The model under review builds one solid part; all positions refer to its coordinate system, in mm. A direction names the side the tool comes from. Round coordinates to 2 decimals unless told otherwise and drop trailing zeros. Write each loop counter-clockwise with the first axis right and the second up, starting at its lowest first coordinate (ties: lowest second). Pieces come first, ordered by that corner, then holes. Notation, with made-up numbers: (51, 79) -> (66, 79) arc R27 ccw to (66, 111) -> close; hole circle Ø3 at (82, 55). An arc over 180 degrees is marked (long way). Return JSON: item names as keys, results as strings. Group by question number.
1. Take a section at C-C, the plane y = -63. Write out the cut boundary in (x, z).
2. Take a section at B-B, the plane x = 33.5. Write out the cut boundary in (y, z), then the cut area to 3 significant figures.
3. Mouldability with a two-part tool opening along X and no side actions: class faces 1 (the flat face through (31, -38, 8.113)), 2 (the flat face through (53, -65, 33.513)), 3 (the flat face through (60.477, -47, 2)) as pulls with the +X half, pulls with the -X half, needs draft (parallel to the pull), parting line crosses it, or undercut.
4. Take a section at A-A, the plane z = 11.5. Write out the cut boundary in (x, y), then the cut area to 3 significant figures.
5. For line 1 along Z through (x, y) = (34, -16.5); line 2 along X through (y, z) = (-61, 18.5); line 3 along Y through (x, z) = (43, 29.5), list the stretches that pass through material, from the lowest coordinate up. Write a range as from..to.
6. Take a section at D-D, the plane x = -11.5. Write out the cut boundary in (y, z).
7. Tool access review of faces 4 (the flat face through (3.45, -38.63, 20.63)), 5 (the flat face through (47.955, -56.883, 20.635)), 6 (the flat face through (-1, 0, 8)): name each direction out of +Z, -Z, +X, -X, +Y, -Y from which nothing blocks a thin tool from reaching the whole face with its end or side.
8. Clearance check with a flat-ended pin moving along its axis: P1, Ø3, axis at x = 35.5, y = -30, coming from the +Z side. State where the tip first meets the part, or that it passes through.
from build123d import *

# Parameters (mm, degrees)
F0_W     = 101.6
F0_H     = 25.4
F1_DEPTH = 76.2
F3_DEPTH = 25.4
F5_DEPTH = 25.4


with BuildPart() as f1:
    # F0 (on Front) → F1 (new body)
    with BuildSketch(Plane.XZ):
        with Locations((9.67671, -4.587205)):
            Rectangle(F0_W, F0_H)
    extrude(amount=F1_DEPTH)

    # F2 (on face) → F3 (join)
    with BuildSketch(Plane.XY.offset(8.112795)):
        Polygon((60.47671, -38.1), (35.07671, -76.2), (60.47671, -76.2), align=None)
    extrude(amount=F3_DEPTH)

    # F4 (on face) → F5 (join)
    with BuildSketch(Plane.XY.offset(8.112795)):
        Polygon((-41.12329, 0), (-41.12329, -76.2), (-14.954321, -76.2), (22.37671, 0), align=None)
    extrude(amount=F5_DEPTH)


solid = f1.part
Output:
{
 "1": {"outline": "(-41.12, -17.29) -> (60.48, -17.29) -> (60.48, 33.51) -> (43.88, 33.51) -> (43.88, 8.11) -> (-8.49, 8.11) -> (-8.49, 33.51) -> (-41.12, 33.51) -> close"},
 "2": {"outline": "(-76.2, -17.29) -> (0, -17.29) -> (0, 8.11) -> (-76.2, 8.11) -> close", "area": "1,940 mm^2"},
 "3": {"face 1": "undercut", "face 2": "needs draft", "face 3": "pulls with the +X half"},
 "4": {"outline": "(-41.12, -76.2) -> (-14.95, -76.2) -> (22.38, 0) -> (-41.12, 0) -> close; (35.08, -76.2) -> (60.48, -76.2) -> (60.48, -38.1) -> close", "area": "3,900 mm^2"},
 "5": {"line 1": "z = -17.29..8.11", "line 2": "x = -41.12..-7.51, 45.21..60.48", "line 3": "y = -76.2..-64.32"},
 "6": {"outline": "(-76.2, -17.29) -> (0, -17.29) -> (0, 33.51) -> (-69.15, 33.51) -> (-69.15, 8.11) -> (-76.2, 8.11) -> close"},
 "7": {"face 4": "+Z, -Y", "face 5": "+Z, +Y", "face 6": "+Z, -Z, +X, -X, +Y"},
 "8": {"P1": "stops at z = 8.11"}
}
